Verification items for the finished model (mm, model axes). Face numbers are marked on the shaded views. A direction names the side the tool comes from. Round coordinates to 2 decimals unless told otherwise and drop trailing zeros. Write each loop counter-clockwise with the first axis right and the second up, starting at its lowest first coordinate (ties: lowest second). Pieces come first, ordered by that corner, then holes.
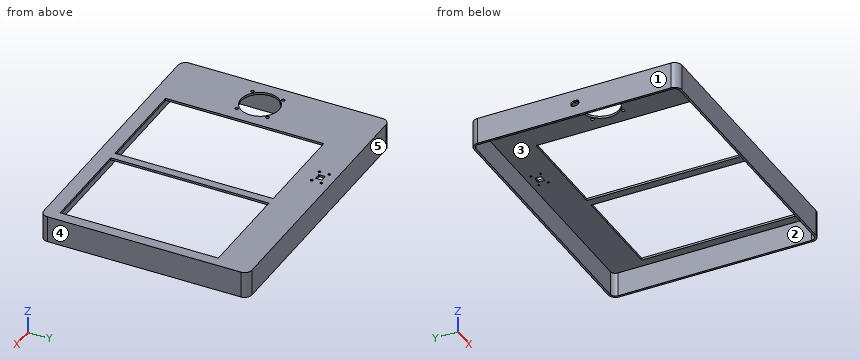
from build123d import *

# Parameters (mm, degrees)
EXTRUDE_1_DEPTH      = 37
SHELL_4_T            = -3
SKETCH_1_8_R         = 2.25
SKETCH_1_8_R_2       = 26.5
SKETCH_1_8_R_3       = 1.25
SKETCH_1_8_W         = 137
SKETCH_1_8_H         = 220
SKETCH_1_8_W_2       = 9
SKETCH_1_8_H_2       = 9
CUT_EXTRUDE_8_DEPTH  = 3
SKETCH_1_9_R         = 1.75
CUT_EXTRUDE_9_DEPTH  = 1.5
CUT_EXTRUDE_10_DEPTH = 3


with BuildPart() as part:
    # 草图1 → 凸台-拉伸1 (new body)
    with BuildSketch(Plane.XY):
        with BuildLine():
            Line((-68, 39.2), (295.5, 39.2))
            ThreePointArc((295.5, 39.2), (302.571067812, 36.271067812), (305.5, 29.2))
            Line((305.5, 29.2), (305.5, -240))
            ThreePointArc((305.5, -240), (302.571067812, -247.071067812), (295.5, -250))
            Line((295.5, -250), (-68, -250))
            ThreePointArc((-68, -250), (-75.071067812, -247.071067812), (-78, -240))
            Line((-78, -240), (-78, 29.2))
            ThreePointArc((-78, 29.2), (-75.071067812, 36.271067812), (-68, 39.2))
        make_face()
    extrude(amount=-EXTRUDE_1_DEPTH)

    # 抽壳4
    shell_4_openings = [part.faces().sort_by_distance(p)[0] for p in [
        (113.75, -105.4, -37),
    ]]
    offset(amount=SHELL_4_T, openings=shell_4_openings, kind=Kind.INTERSECTION)

    # 草图1<8> → 切除-拉伸8 (cut)
    with BuildSketch(Plane.XY):
        with Locations((-58, -98.5)):
            Circle(SKETCH_1_8_R)
        with Locations((-36.5, -120)):
            Circle(SKETCH_1_8_R_2)
        with Locations((-15, -98.5)):
            Circle(SKETCH_1_8_R)
        with Locations((-15, -141.5)):
            Circle(SKETCH_1_8_R)
        with Locations((-58, -141.5)):
            Circle(SKETCH_1_8_R)
        with Locations((62.85, 27.2)):
            Circle(SKETCH_1_8_R_3)
        with Locations((84.15, 27.2)):
            Circle(SKETCH_1_8_R_3)
        with Locations((84.15, 13.9)):
            Circle(SKETCH_1_8_R_3)
        with Locations((62.85, 13.9)):
            Circle(SKETCH_1_8_R_3)
        with Locations((73.5, -120)):
            Rectangle(SKETCH_1_8_W, SKETCH_1_8_H)
        with Locations((222, -120)):
            Rectangle(SKETCH_1_8_W, SKETCH_1_8_H)
        with Locations((73.5, 20.5)):
            Rectangle(SKETCH_1_8_W_2, SKETCH_1_8_H_2)
    extrude(amount=-CUT_EXTRUDE_8_DEPTH, mode=Mode.SUBTRACT)

    # 草图1<9> → 切除-拉伸9 (cut)
    with BuildSketch(Plane.XY):
        with Locations((62.85, 27.2)):
            Circle(SKETCH_1_9_R)
        with Locations((84.15, 27.2)):
            Circle(SKETCH_1_9_R)
        with Locations((84.15, 13.9)):
            Circle(SKETCH_1_9_R)
        with Locations((62.85, 13.9)):
            Circle(SKETCH_1_9_R)
    extrude(amount=-CUT_EXTRUDE_9_DEPTH, mode=Mode.SUBTRACT)

    # 草图2 → 切除-拉伸10 (cut)
    with BuildSketch(Plane.ZY.offset(78)):
        with BuildLine():
            Line((-19.5, -100.8), (-18.5, -100.8))
            ThreePointArc((-18.5, -100.8), (-16.025126266, -101.825126266), (-15, -104.3))
            Line((-15, -104.3), (-15, -108.3))
            ThreePointArc((-15, -108.3), (-16.025126266, -110.774873734), (-18.5, -111.8))
            Line((-18.5, -111.8), (-19.5, -111.8))
            ThreePointArc((-19.5, -111.8), (-21.974873734, -110.774873734), (-23, -108.3))
            Line((-23, -108.3), (-23, -104.3))
            ThreePointArc((-23, -104.3), (-21.974873734, -101.825126266), (-19.5, -100.8))
        make_face()
    extrude(amount=-CUT_EXTRUDE_10_DEPTH, mode=Mode.SUBTRACT)


solid = part.part
Q1. Sectioned sample at B-B (y = -46). Enter the section's corners in (x, z).
Recorded:
outline: (-78, -37) - (-75, -37) - (-75, -3) - (5, -3) - (5, 0) - (-78, 0) - close; (142, -3) - (153.5, -3) - (153.5, 0) - (142, 0) - close; (290.5, -3) - (302.5, -3) - (302.5, -37) - (305.5, -37) - (305.5, 0) - (290.5, 0) - close
Q2. Tool access check on the marked faces 1 and 2. Record the directions out of +Z, -Z, +X, -X, +Y, -Y that give a thin tool (end or side, any length) a straight path to the whole face; none if there is none.
Recorded:
face 1: +Z, -Z, -X, +Y, -Y
face 2: -Z
Q3. Depth check by flat-ended pin: P1, Ø2, axis at x = 62.85, y = 27.2, coming from the +Z side; P2, Ø0.5, axis at x = -76.5, z = -19, coming from the -Y side; P3, Ø0.5, axis at x = -77, z = -19, coming from the +Y side; P4, Ø3, axis at x = 84.15, y = 27.2, coming from the -Z side. Enter the tip coordinate at first touch or a pass-through.
Recorded:
P1: passes through
P2: stops at y = -245.65
P3: stops at y = 34.04
P4: stops at z = -3
Q4. Release check for a two-part mould opening along Y. For the marked faces 3, 4 and 5 record: released by +Y, released by -Y, zero draft, split by the parting line, or undercut.
Recorded:
face 3: undercut
face 4: zero draft
face 5: released by +Y
Q5. Material ranges on line 1 along Y through (x, z) = (84.15, -2.6); line 2 along Y through (x, z) = (84.15, -0.35); line 3 along Y through (x, z) = (94, -21), recorded low to high.
Recorded:
line 1: y = -250 to -230, -10 to 12.65, 15.15 to 25.95, 28.45 to 39.2
line 2: y = -250 to -230, -10 to 12.15, 15.65 to 25.45, 28.95 to 39.2
line 3: y = -250 to -247, 36.2 to 39.2
Q6. Sectioned sample at C-C (y = -120). Enter the section's corners in (x, z), plus the area to 4 significant figures.
Recorded:
outline: (-78, -37) - (-75, -37) - (-75, -3) - (-63, -3) - (-63, 0) - (-78, 0) - close; (-10, -3) - (5, -3) - (5, 0) - (-10, 0) - close; (142, -3) - (153.5, -3) - (153.5, 0) - (142, 0) - close; (290.5, -3) - (302.5, -3) - (302.5, -37) - (305.5, -37) - (305.5, 0) - (290.5, 0) - close
area: 373.5 mm2
Q7. Sectioned sample at D-D (x = -36.5). Enter the section's corners in (y, z), plus the area to 3 significant figures.
Recorded:
outline: (-250, -37) - (-247, -37) - (-247, -3) - (-146.5, -3) - (-146.5, 0) - (-250, 0) - close; (-93.5, -3) - (36.2, -3) - (36.2, -37) - (39.2, -37) - (39.2, 0) - (-93.5, 0) - close
area: 913 mm2
Q8. Sectioned sample at A-A (x = 203). Enter the section's corners in (y, z).
Recorded:
outline: (-250, -37) - (-247, -37) - (-247, -3) - (-230, -3) - (-230, 0) - (-250, 0) - close; (-10, -3) - (36.2, -3) - (36.2, -37) - (39.2, -37) - (39.2, 0) - (-10, 0) - close
